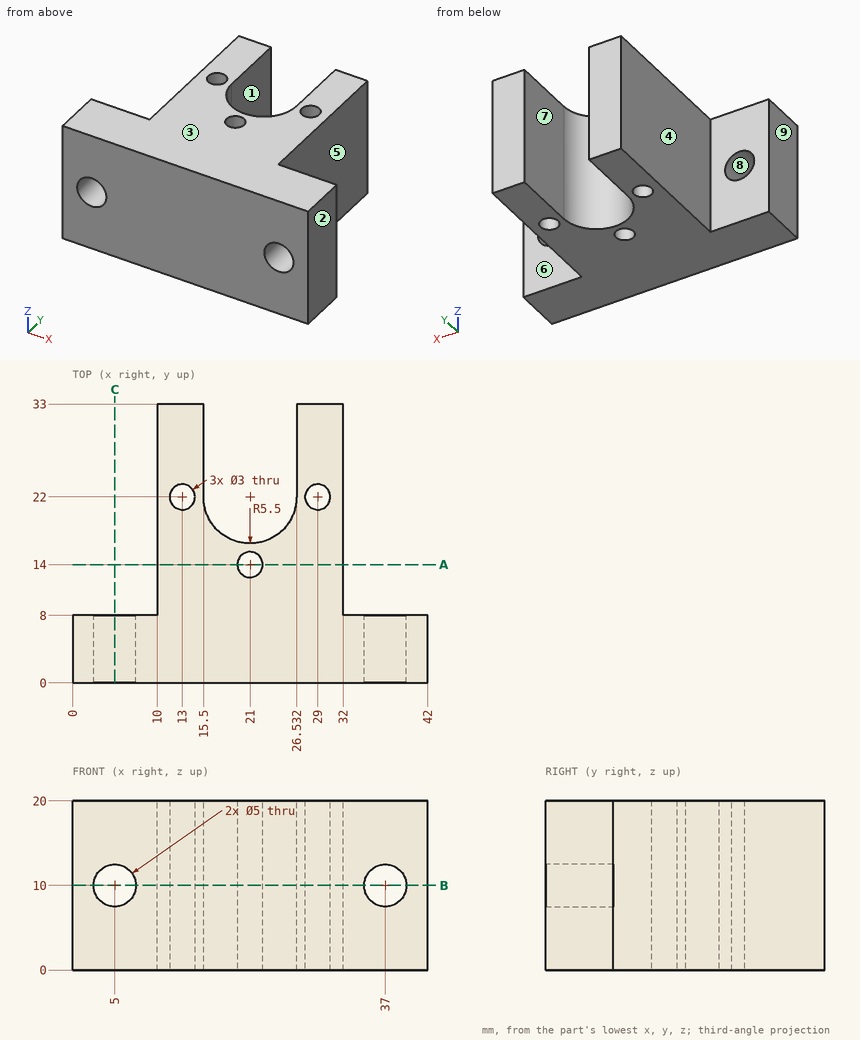
Check sheet for the drawn part. Datum: minimum x, y, z corner. Units: mm. A direction names the side the tool comes from. Give positions to 0.01 mm unless a question says otherwise; leave off trailing zeros. Order: outer loops, then holes, each group sorted by start corner. A loop starts at its lowest first (then second) coordinate and runs counter-clockwise, first axis right, second up. Notation, with made-up numbers: (9.25, 80) -> (32.25, 80) arc R27 ccw to (32.25, 100) -> close; hole circle Ø11 at (-7.5, -13.75). An arc over 180 degrees is marked (long way). Return JSON: item names as keys, results as strings.
1. Cross-section at C-C, the plane x = 5. Record the cut outline in (y, z), plus the area to 3 significant figures.
From the geometry:
{"outline": "(0, 0) -> (8, 0) -> (8, 7.5) -> (0, 7.5) -> close; (0, 12.5) -> (8, 12.5) -> (8, 20) -> (0, 20) -> close", "area": "120 mm^2"}
2. Set-up check for the marked faces 1, 2, 3, 4 and 5: record each of +Z, -Z, +X, -X, +Y, -Y from which the full face is reachable in a straight line by a thin tool's end or side.
From the geometry:
{"face 1": "+Z, -Z, +Y", "face 2": "+Z, -Z, +X, +Y, -Y", "face 3": "+Z, +X, -X, +Y, -Y", "face 4": "+Z, -Z, -X, +Y", "face 5": "+Z, -Z, +X, +Y"}
3. Cross-section at B-B, the plane z = 10. Count the separate pieces of the cut face and the enclosed holes in it, plus the area to 3 significant figures.
From the geometry:
{"separate pieces": "3", "enclosed holes": "3", "area": "616 mm^2"}
4. Mould release check, pull along X, two halves, no side actions. Record for the marked faces 6, 7, 8 and 9: +X half, -X half, draft (parallel to the pull), parting line (faces both ways), or undercut.
From the geometry:
{"face 6": "draft", "face 7": "undercut", "face 8": "undercut", "face 9": "-X half"}
5. Cross-section at A-A, the plane y = 14. Record the cut outline in (x, z), plus the area to 3 significant figures.
From the geometry:
{"outline": "(10, 0) -> (19.5, 0) -> (19.5, 20) -> (10, 20) -> close; (22.5, 0) -> (32, 0) -> (32, 20) -> (22.5, 20) -> close", "area": "380 mm^2"}
6. Material ranges on probe 1 along X at (y, z) = (6, 10); probe 2 along Y at (x, z) = (21, 10.25); probe 3 along Y at (x, z) = (29, 6.25), recorded low to high. Write a range as [from, to].
From the geometry:
{"probe 1": "[0, 2.5], [7.5, 34.5], [39.5, 42]", "probe 2": "[0, 12.5], [15.5, 16.5]", "probe 3": "[0, 20.5], [23.5, 33]"}
7. Go/stop test with flat-tipped pins: P1, Ø1.8, axis at x = 29, y = 22, coming from the -Z side; P2, Ø10, axis at y = 9.5, z = 13, coming from the +X side; P3, Ø1.5, axis at y = 11, z = 17, coming from the -X side; P4, Ø5.5, axis at y = 29.5, z = 11, coming from the +X side. Record where each tip stops, or that it passes through.
From the geometry:
{"P1": "through", "P2": "x = 42", "P3": "x = 10", "P4": "x = 32"}
